```python
from build123d import *

# Parameters (mm, degrees)
F0_R     = 2.5
F1_DEPTH = 4
F2_R     = 5


with BuildPart() as f1:
    # F0 (on Top) → F1 (new body)
    with BuildSketch(Plane.XY):
        with BuildLine():
            ThreePointArc((-20, -20), (0, -18), (20, -20))
            ThreePointArc((20, -20), (18, 0), (20, 20))
            ThreePointArc((20, 20), (0, 18), (-20, 20))
            ThreePointArc((-20, 20), (-18, 0), (-20, -20))
        make_face()
        with BuildLine():
            ThreePointArc((16.5, 14), (15.767766953, 12.232233047), (14, 11.5))
            Line((14, 11.5), (14, -11.5))
            ThreePointArc((14, -11.5), (15.767766953, -12.232233047), (16.5, -14))
            ThreePointArc((16.5, -14), (14, -16.5), (11.5, -14))
            Line((11.5, -14), (-11.5, -14))
            ThreePointArc((-11.5, -14), (-15.767766953, -15.767766953), (-14, -11.5))
            Line((-14, -11.5), (-14, 11.5))
            ThreePointArc((-14, 11.5), (-15.767766953, 15.767766953), (-11.5, 14))
            Line((-11.5, 14), (11.5, 14))
            ThreePointArc((11.5, 14), (14, 16.5), (16.5, 14))
        make_face(mode=Mode.SUBTRACT)
        with BuildLine():
            Line((14, -11.5), (14, 11.5))
            ThreePointArc((14, 11.5), (12.232233047, 12.232233047), (11.5, 14))
            Line((11.5, 14), (-11.5, 14))
            ThreePointArc((-11.5, 14), (-12.232233047, 12.232233047), (-14, 11.5))
            Line((-14, 11.5), (-14, -11.5))
            ThreePointArc((-14, -11.5), (-12.232233047, -12.232233047), (-11.5, -14))
            Line((-11.5, -14), (11.5, -14))
            ThreePointArc((11.5, -14), (12.232233047, -12.232233047), (14, -11.5))
        make_face()
        with BuildLine():
            Line((2.5, -7.5), (-2.5, -7.5))
            ThreePointArc((-2.5, -7.5), (-11.0355339059, -11.0355339059), (-7.5, -2.5))
            Line((-7.5, -2.5), (-7.5, 2.5))
            ThreePointArc((-7.5, 2.5), (-11.0355339059, 11.0355339059), (-2.5, 7.5))
            Line((-2.5, 7.5), (2.5, 7.5))
            ThreePointArc((2.5, 7.5), (7.5, 12.5), (12.5, 7.5))
            ThreePointArc((12.5, 7.5), (11.0355339059, 3.9644660941), (7.5, 2.5))
            Line((7.5, 2.5), (7.5, -2.5))
            ThreePointArc((7.5, -2.5), (11.0355339059, -3.9644660941), (12.5, -7.5))
            ThreePointArc((12.5, -7.5), (7.5, -12.5), (2.5, -7.5))
        make_face(mode=Mode.SUBTRACT)
        with BuildLine():
            ThreePointArc((-7.5, -2.5), (-3.9644660941, -3.9644660941), (-2.5, -7.5))
            Line((-2.5, -7.5), (2.5, -7.5))
            ThreePointArc((2.5, -7.5), (3.9644660941, -3.9644660941), (7.5, -2.5))
            Line((7.5, -2.5), (7.5, 2.5))
            ThreePointArc((7.5, 2.5), (3.9644660941, 3.9644660941), (2.5, 7.5))
            Line((2.5, 7.5), (-2.5, 7.5))
            ThreePointArc((-2.5, 7.5), (-3.9644660941, 3.9644660941), (-7.5, 2.5))
            Line((-7.5, 2.5), (-7.5, -2.5))
        make_face()
        Circle(F0_R, mode=Mode.SUBTRACT)
        with BuildLine():
            Line((-7.5, 5.5), (-7.5, 2.5))
            ThreePointArc((-7.5, 2.5), (-3.9644660941, 3.9644660941), (-2.5, 7.5))
            Line((-2.5, 7.5), (-5.5, 7.5))
            ThreePointArc((-5.5, 7.5), (-6.0857864376, 6.0857864376), (-7.5, 5.5))
        make_face()
        with BuildLine():
            ThreePointArc((-2.5, 7.5), (-11.0355339059, 11.0355339059), (-7.5, 2.5))
            Line((-7.5, 2.5), (-7.5, 5.5))
            ThreePointArc((-7.5, 5.5), (-8.9142135624, 8.9142135624), (-5.5, 7.5))
            Line((-5.5, 7.5), (-2.5, 7.5))
        make_face()
        with BuildLine():
            Line((7.5, 5.5), (7.5, 2.5))
            ThreePointArc((7.5, 2.5), (11.0355339059, 3.9644660941), (12.5, 7.5))
            ThreePointArc((12.5, 7.5), (7.5, 12.5), (2.5, 7.5))
            Line((2.5, 7.5), (5.5, 7.5))
            ThreePointArc((5.5, 7.5), (7.5, 9.5), (9.5, 7.5))
            ThreePointArc((9.5, 7.5), (8.9142135624, 6.0857864376), (7.5, 5.5))
        make_face()
        with BuildLine():
            ThreePointArc((2.5, 7.5), (3.9644660941, 3.9644660941), (7.5, 2.5))
            Line((7.5, 2.5), (7.5, 5.5))
            ThreePointArc((7.5, 5.5), (6.0857864376, 6.0857864376), (5.5, 7.5))
            Line((5.5, 7.5), (2.5, 7.5))
        make_face()
        with BuildLine():
            ThreePointArc((-7.5, -2.5), (-11.0355339059, -11.0355339059), (-2.5, -7.5))
            Line((-2.5, -7.5), (-5.5, -7.5))
            ThreePointArc((-5.5, -7.5), (-8.9142135624, -8.9142135624), (-7.5, -5.5))
            Line((-7.5, -5.5), (-7.5, -2.5))
        make_face()
        with BuildLine():
            Line((5.5, -7.5), (2.5, -7.5))
            ThreePointArc((2.5, -7.5), (7.5, -12.5), (12.5, -7.5))
            ThreePointArc((12.5, -7.5), (11.0355339059, -3.9644660941), (7.5, -2.5))
            Line((7.5, -2.5), (7.5, -5.5))
            ThreePointArc((7.5, -5.5), (8.9142135624, -6.0857864376), (9.5, -7.5))
            ThreePointArc((9.5, -7.5), (7.5, -9.5), (5.5, -7.5))
        make_face()
        with BuildLine():
            ThreePointArc((7.5, -2.5), (3.9644660941, -3.9644660941), (2.5, -7.5))
            Line((2.5, -7.5), (5.5, -7.5))
            ThreePointArc((5.5, -7.5), (6.0857864376, -6.0857864376), (7.5, -5.5))
            Line((7.5, -5.5), (7.5, -2.5))
        make_face()
        with BuildLine():
            Line((-5.5, -7.5), (-2.5, -7.5))
            ThreePointArc((-2.5, -7.5), (-3.9644660941, -3.9644660941), (-7.5, -2.5))
            Line((-7.5, -2.5), (-7.5, -5.5))
            ThreePointArc((-7.5, -5.5), (-6.0857864376, -6.0857864376), (-5.5, -7.5))
        make_face()
    extrude(amount=F1_DEPTH)

    # F2
    f2_edges = [f1.edges().sort_by_distance(p)[0] for p in [
        (20, -20, 2),
        (20, 20, 2),
        (-20, -20, 2),
        (-20, 20, 2),
    ]]
    fillet(f2_edges, radius=F2_R)


solid = f1.part
```
Model file for the job. Use its own axes, mm. Round coordinates to 2 decimals unless told otherwise and drop trailing zeros. Write each loop counter-clockwise with the first axis right and the second up, starting at its lowest first coordinate (ties: lowest second). Pieces come first, ordered by that corner, then holes. Notation, with made-up numbers: (49, -33) - (64, -33) arc R7 cw to (64, -26) - close; hole circle Ø3 at (82.5, -37). An arc over 180 degrees is marked (long way). Use CSV: the item, a comma, the result in double quotes. Start each with the question number.
Item 1: Band-saw the part on A-A (y = 0). Write the cut outline in (x, z), and give its area (3 significant figures).
Item 2: Pin check, flat tips, straight feed: P1, Ø1.5, axis at x = 15, z = 3, coming from the -Y side; P2, Ø3, axis at x = 0, y = 0, coming from the +Z side; P3, Ø2, axis at x = -2.5, z = 3, coming from the +Y side. Stop position of each tip, or through.
Item 3: Drill centre lines: L1, parallel to Y at x = -14, z = 1.65; L2, parallel to Y at x = -13, z = 3.6; L3, parallel to X at y = 7.5, z = 1.4. Where is each one in solid material? Low to high. Write a range as [from, to].
Item 4: Band-saw the part on C-C (x = 12.5). Write the cut outline in (y, z), and give its area (3 significant figures).
Item 5: Two-plate mould, pull along X, no slides. Class faces 1 (the face through (4, 0, 4)), 2 (the face through (0, 18, 2)), 3 (the face through (18, 0, 2)): released by +X, released by -X, zero draft, split by the parting line, or undercut.
Checked values:
1,outline,"(-18, 0) - (-2.5, 0) - (-2.5, 4) - (-18, 4) - close; (2.5, 0) - (18, 0) - (18, 4) - (2.5, 4) - close"
1,area,"124 mm²"
2,P1,"stops at y = -18.91"
2,P2,"passes through"
2,P3,"stops at y = 18.06"
3,L1,"y = [-18.92, -16.5], [-11.5, 11.5], [16.5, 18.92]"
3,L2,"y = [-18.84, -16.29], [-11.71, 11.71], [16.29, 18.84]"
3,L3,"x = [-18.28, -9.5], [-5.5, 5.5], [9.5, 18.28]"
4,outline,"(-18.78, 0) - (-16, 0) - (-16, 4) - (-18.78, 4) - close; (-12, 0) - (12, 0) - (12, 4) - (-12, 4) - close; (16, 0) - (18.78, 0) - (18.78, 4) - (16, 4) - close"
4,area,"118 mm²"
5,face 1,"zero draft"
5,face 2,"undercut"
5,face 3,"released by +X"
